Autodesk Fusion 360 part; units mm, degrees
sketch "Sketch1" plane through (0, 0, 0) normal (0, 0, 1) x (1, 0, 0)
  line L0 (-250, 100) -> (250, 100)
  line L1 (250, 100) -> (250, -100)
  line L2 (250, -100) -> (-250, -100)
  line L3 (-250, -100) -> (-250, 100)
  line L4 (0, 100) -> (0, -100) construction
  line L5 (-250, 0) -> (250, 0) construction
  circle A0 centre (0, 0) radius 20
  circle A1 centre (0, 0) radius 10
  dimension "Total_Height" = 200
  dimension "Total_Width" = 500
  dimension "Inner_Radius" = 10
  dimension "Outer_Radius" = 20
extrude "Extrude1" add sketch "Sketch1" along normal mid plane 10 contours L0 L1 L2 L3
extrude "Extrude2" add sketch "Sketch1" along normal mid plane 30 contours A0
fillet "Fillet1" radius 5 2 edges at (-18.6465, 7.2323, 5) (-18.6465, -7.2323, -5)
Check sheet for the modelled part. Datum: model origin and axes. Units: mm. A direction names the side the tool comes from. Give positions to 0.01 mm unless a question says otherwise; leave off trailing zeros. Loops run counter-clockwise (first coordinate to the right, second up) from the corner with the lowest first, then second, coordinate; pieces in that order, holes last. Notation, with made-up numbers: (76, -34) - (130, -34) arc R16 ccw to (130, -29) - close; hole circle Ø10 at (-17.75, -17.5). An arc over 180 degrees is marked (long way). One line per question, with ' | ' between items. Start each with the question number.
1. Cross-section at A-A, the plane y = 0. Enter the section's corners in (x, z), plus the area to 3 significant figures.
2. Gauge pin test, flat ends, axial feed: pin 1 Ø6 at (x, y) = (171.5, -1.5) entering from +Z; pin 2 Ø1.5 at (x, y) = (77, 61.5) entering from -Z; pin 3 Ø10 at (y, z) = (60, 9.5) entering from -X; pin 4 Ø8 at (y, z) = (7, -10) entering from -X. Record the tip position at first contact, or that the pin passes through.
3. Cross-section at B-B, the plane x = 0. Enter the section's corners in (y, z), plus the area to 3 significant figures.
4. Cross-section at D-D, the plane y = -64. Enter the section's corners in (x, z).
5. Set-up check for faces 1 (the flat face through (250, 1, 0)), 2 (the cylindrical face through (-4.336, 19.524, 12.465)): record each of +Z, -Z, +X, -X, +Y, -Y from which the full face is reachable in a straight line by a thin tool's end or side.
6. Draft check along Y on faces 3 (the flat face through (-3, 46, -5)), 4 (the cylindrical face through (-2.17, 9.76, -0.21)), 5 (the cylindrical face through (-4.336, -19.524, -12.465)), 6 (the flat face through (-3, 100, 0)). Enter one of: released by +Y, released by -Y, zero draft, split by the parting line, or undercut.
7. Cross-section at C-C, the plane x = -141. Enter the section's corners in (y, z), plus the area to 3 significant figures.
8. Material ranges on line 1 along Y through (x, z) = (0, 1); line 2 along Z through (x, y) = (137, -15.5); line 3 along Y through (x, z) = (8, 3.5), recorded low to high. Write a range as [from, to].
Check result:
1) outline: (-250, -5) - (-25, -5) arc R5 cw to (-20, -10) - (-20, -15) - (-10, -15) - (-10, 15) - (-20, 15) - (-20, 10) arc R5 cw to (-25, 5) - (-250, 5) - close; (10, -15) - (20, -15) - (20, -10) arc R5 cw to (25, -5) - (250, -5) - (250, 5) - (25, 5) arc R5 cw to (20, 10) - (20, 15) - (10, 15) - close | area: 5,220 mm2
2) pin 1: stops at z = 5 | pin 2: stops at z = -5 | pin 3: stops at x = -250 | pin 4: stops at x = -21
3) outline: (-100, -5) - (-25, -5) arc R5 cw to (-20, -10) - (-20, -15) - (-10, -15) - (-10, 15) - (-20, 15) - (-20, 10) arc R5 cw to (-25, 5) - (-100, 5) - close; (10, -15) - (20, -15) - (20, -10) arc R5 cw to (25, -5) - (100, -5) - (100, 5) - (25, 5) arc R5 cw to (20, 10) - (20, 15) - (10, 15) - close | area: 2,220 mm2
4) outline: (-250, -5) - (250, -5) - (250, 5) - (-250, 5) - close
5) face 1: +Z, -Z, +X, +Y, -Y | face 2: +Z
6) face 3: zero draft | face 4: undercut | face 5: split by the parting line | face 6: released by +Y
7) outline: (-100, -5) - (100, -5) - (100, 5) - (-100, 5) - close | area: 2,000 mm2
8) line 1: y = [-100, -10], [10, 100] | line 2: z = [-5, 5] | line 3: y = [-100, -6], [6, 100]
